from build123d import *

# Parameters (mm, degrees)
F0_R     = 2.5
F1_DEPTH = 3
F2_DEPTH = 5
F3_R     = 3
F3_R_2   = 2.5
F4_DEPTH = 2


with BuildPart() as f1:
    # F0 (on Top) → F1 (new body)
    with BuildSketch(Plane.XY):
        with BuildLine():
            Line((-28, 0), (0, 0))
            Line((0, 0), (0, 25))
            Line((0, 25), (-13, 25))
            ThreePointArc((-13, 25), (-16.3893239512, 24.6120663547), (-19.6033368631, 23.4683310871))
            ThreePointArc((-19.6033368631, 23.4683310871), (-18.0971524178, 22.6214718865), (-17.5, 21))
            ThreePointArc((-17.5, 21), (-20.3463811518, 18.5241122607), (-22.4040160781, 21.6860806776))
            ThreePointArc((-22.4040160781, 21.6860806776), (-25.1440747457, 18.8046265435), (-27.0307720104, 15.3044732813))
            ThreePointArc((-27.0307720104, 15.3044732813), (-25.9175651302, 14.3832805258), (-25.5, 13))
            ThreePointArc((-25.5, 13), (-26.2292882388, 11.235182769), (-27.991663887, 10.5000138982))
            ThreePointArc((-27.991663887, 10.5000138982), (-27.997915827, 10.2500416911), (-28, 10))
            Line((-28, 10), (-28, 7.5))
            ThreePointArc((-28, 7.5), (-26.232233047, 6.767766953), (-25.5, 5))
            ThreePointArc((-25.5, 5), (-26.232233047, 3.232233047), (-28, 2.5))
            Line((-28, 2.5), (-28, 0))
        make_face()
        with Locations((-20, 5)):
            Circle(F0_R, mode=Mode.SUBTRACT)
        with Locations((-12, 5)):
            Circle(F0_R, mode=Mode.SUBTRACT)
        with Locations((-4, 5)):
            Circle(F0_R, mode=Mode.SUBTRACT)
        with Locations((-20, 13)):
            Circle(F0_R, mode=Mode.SUBTRACT)
        with Locations((-12, 13)):
            Circle(F0_R, mode=Mode.SUBTRACT)
        with Locations((-4, 13)):
            Circle(F0_R, mode=Mode.SUBTRACT)
        with Locations((-12, 21)):
            Circle(F0_R, mode=Mode.SUBTRACT)
        with Locations((-4, 21)):
            Circle(F0_R, mode=Mode.SUBTRACT)
        with BuildLine():
            ThreePointArc((-17.5, 21), (-18.0971524178, 22.6214718865), (-19.6033368631, 23.4683310871))
            ThreePointArc((-19.6033368631, 23.4683310871), (-21.0531323829, 22.654922316), (-22.4040160781, 21.6860806776))
            ThreePointArc((-22.4040160781, 21.6860806776), (-20.3463811518, 18.5241122607), (-17.5, 21))
        make_face()
        with BuildLine():
            Line((0, 25), (0, 0))
            Line((0, 0), (28, 0))
            Line((28, 0), (28, 2.5))
            ThreePointArc((28, 2.5), (25.5, 5), (28, 7.5))
            Line((28, 7.5), (28, 10))
            ThreePointArc((28, 10), (27.997915827, 10.2500416911), (27.991663887, 10.5000138982))
            ThreePointArc((27.991663887, 10.5000138982), (25.5485483108, 12.5097096622), (27.0307720104, 15.3044732813))
            ThreePointArc((27.0307720104, 15.3044732813), (25.1440747457, 18.8046265435), (22.4040160781, 21.6860806776))
            ThreePointArc((22.4040160781, 21.6860806776), (22.4758877393, 21.3463811518), (22.5, 21))
            ThreePointArc((22.5, 21), (18.3785281135, 19.0971524178), (19.6033368631, 23.4683310871))
            ThreePointArc((19.6033368631, 23.4683310871), (16.3893239512, 24.6120663547), (13, 25))
            Line((13, 25), (0, 25))
        make_face()
        with Locations((4, 5)):
            Circle(F0_R, mode=Mode.SUBTRACT)
        with Locations((12, 5)):
            Circle(F0_R, mode=Mode.SUBTRACT)
        with Locations((20, 5)):
            Circle(F0_R, mode=Mode.SUBTRACT)
        with Locations((4, 13)):
            Circle(F0_R, mode=Mode.SUBTRACT)
        with Locations((12, 13)):
            Circle(F0_R, mode=Mode.SUBTRACT)
        with Locations((20, 13)):
            Circle(F0_R, mode=Mode.SUBTRACT)
        with Locations((4, 21)):
            Circle(F0_R, mode=Mode.SUBTRACT)
        with Locations((12, 21)):
            Circle(F0_R, mode=Mode.SUBTRACT)
        with BuildLine():
            ThreePointArc((22.4040160781, 21.6860806776), (21.0531323829, 22.654922316), (19.6033368631, 23.4683310871))
            ThreePointArc((19.6033368631, 23.4683310871), (18.3785281135, 19.0971524178), (22.5, 21))
            ThreePointArc((22.5, 21), (22.4758877393, 21.3463811518), (22.4040160781, 21.6860806776))
        make_face()
        with BuildLine():
            ThreePointArc((-27.0307720104, 15.3044732813), (-27.7087101354, 12.9417420271), (-27.991663887, 10.5000138982))
            ThreePointArc((-27.991663887, 10.5000138982), (-26.2292882388, 11.235182769), (-25.5, 13))
            ThreePointArc((-25.5, 13), (-25.9175651302, 14.3832805258), (-27.0307720104, 15.3044732813))
        make_face()
        with BuildLine():
            Line((-28, 7.5), (-28, 2.5))
            ThreePointArc((-28, 2.5), (-26.232233047, 3.232233047), (-25.5, 5))
            ThreePointArc((-25.5, 5), (-26.232233047, 6.767766953), (-28, 7.5))
        make_face()
        with BuildLine():
            ThreePointArc((28, 7.5), (25.5, 5), (28, 2.5))
            Line((28, 2.5), (28, 7.5))
        make_face()
        with BuildLine():
            ThreePointArc((27.991663887, 10.5000138982), (27.7087101354, 12.9417420271), (27.0307720104, 15.3044732813))
            ThreePointArc((27.0307720104, 15.3044732813), (25.5485483108, 12.5097096622), (27.991663887, 10.5000138982))
        make_face()
    extrude(amount=F1_DEPTH)

    # F0 (on Top) → F2 (join)
    with BuildSketch(Plane.XY):
        with Locations((-20, 13)):
            Circle(F0_R)
        with Locations((-20, 5)):
            Circle(F0_R)
        with Locations((-12, 5)):
            Circle(F0_R)
        with Locations((-12, 13)):
            Circle(F0_R)
        with Locations((-12, 21)):
            Circle(F0_R)
        with Locations((-4, 21)):
            Circle(F0_R)
        with Locations((-4, 13)):
            Circle(F0_R)
        with Locations((-4, 5)):
            Circle(F0_R)
        with Locations((4, 13)):
            Circle(F0_R)
        with Locations((4, 21)):
            Circle(F0_R)
        with Locations((4, 5)):
            Circle(F0_R)
        with Locations((12, 5)):
            Circle(F0_R)
        with Locations((12, 13)):
            Circle(F0_R)
        with Locations((12, 21)):
            Circle(F0_R)
        with Locations((20, 13)):
            Circle(F0_R)
        with Locations((20, 5)):
            Circle(F0_R)
    extrude(amount=F2_DEPTH)

    # F3 (on Top) → F4 (cut)
    with BuildSketch(Plane.XY):
        with BuildLine():
            Line((13, 23.5), (0, 23.5))
            Line((0, 23.5), (-13, 23.5))
            ThreePointArc((-13, 23.5), (-15.5473326534, 23.2574920838), (-18.0031470352, 22.5386809412))
            ThreePointArc((-18.0031470352, 22.5386809412), (-20.2891608484, 21.3630160664), (-22.3108832056, 19.7753492997))
            ThreePointArc((-22.3108832056, 19.7753492997), (-25.4086043388, 15.3175688394), (-26.5, 10))
            Line((-26.5, 10), (-26.5, 1.5))
            Line((-26.5, 1.5), (0, 1.5))
            Line((0, 1.5), (26.5, 1.5))
            Line((26.5, 1.5), (26.5, 7.3416876048))
            ThreePointArc((26.5, 7.3416876048), (21.0000404053, 8.9844298396), (26.4826520886, 10.6841729742))
            ThreePointArc((26.4826520886, 10.6841729742), (25.26982822, 15.6303921225), (22.3108832056, 19.7753492997))
            ThreePointArc((22.3108832056, 19.7753492997), (20.2891608484, 21.3630160664), (18.0031470352, 22.5386809412))
            ThreePointArc((18.0031470352, 22.5386809412), (15.5473326534, 23.2574920838), (13, 23.5))
        make_face()
        with Locations((-16, 9)):
            Circle(F3_R, mode=Mode.SUBTRACT)
        with Locations((-8, 9)):
            Circle(F3_R, mode=Mode.SUBTRACT)
        with Locations((0, 9)):
            Circle(F3_R, mode=Mode.SUBTRACT)
        with Locations((8, 9)):
            Circle(F3_R, mode=Mode.SUBTRACT)
        with Locations((16, 9)):
            Circle(F3_R, mode=Mode.SUBTRACT)
        with Locations((-16, 17)):
            Circle(F3_R, mode=Mode.SUBTRACT)
        with Locations((-8, 17)):
            Circle(F3_R, mode=Mode.SUBTRACT)
        with Locations((0, 17)):
            Circle(F3_R, mode=Mode.SUBTRACT)
        with Locations((8, 17)):
            Circle(F3_R, mode=Mode.SUBTRACT)
        with Locations((16, 17)):
            Circle(F3_R, mode=Mode.SUBTRACT)
        with BuildLine():
            ThreePointArc((26.5, 10), (26.4956623253, 10.342196438), (26.4826520886, 10.6841729742))
            ThreePointArc((26.4826520886, 10.6841729742), (21.0000404053, 8.9844298396), (26.5, 7.3416876048))
            Line((26.5, 7.3416876048), (26.5, 9))
            Line((26.5, 9), (26.5, 10))
        make_face()
        with Locations((24, 9)):
            Circle(F3_R_2, mode=Mode.SUBTRACT)
        with Locations((16, 9)):
            Circle(F3_R_2)
        with Locations((8, 9)):
            Circle(F3_R_2)
        with Locations((8, 17)):
            Circle(F3_R_2)
        with Locations((16, 17)):
            Circle(F3_R_2)
        with Locations((0, 9)):
            Circle(F3_R_2)
        with Locations((-8, 9)):
            Circle(F3_R_2)
        with Locations((-16, 9)):
            Circle(F3_R_2)
        with Locations((-16, 17)):
            Circle(F3_R_2)
        with Locations((-8, 17)):
            Circle(F3_R_2)
        with Locations((0, 17)):
            Circle(F3_R_2)
        with Locations((24, 9)):
            Circle(F3_R_2)
    extrude(amount=F4_DEPTH, mode=Mode.SUBTRACT)


solid = f1.part
The listing builds one solid part. Answer for the finished solid, in the listing's coordinates (mm). A direction names the side the tool comes from. Coordinates: 2 decimals unless noted, no trailing zeros. Loops run counter-clockwise (first coordinate to the right, second up) from the corner with the lowest first, then second, coordinate; pieces in that order, holes last.
1) Find section A-A on z = 4. Give the number of separate pieces and of enclosed holes in the cut face, then the cut area to 3 significant figures.
2) Determine the mould class of faces 1 (the face through (-2.66, 23.11, 3.99)), 2 (the face through (6, 19, 0)) for opening direction Y: pulls with the +Y half, pulls with the -Y half, needs draft (parallel to the pull), parting line crosses it, or undercut.
3) Flat-ended cylindrical pins translate along their axes: pin 1 Ø1 at (y, z) = (15.5, 2) entering from +X; pin 2 Ø3 at (x, y) = (-16, 17) entering from -Z; pin 3 Ø1 at (y, z) = (20.5, 2) entering from +X. Find the tip coordinate at first contact, or state that the pin passes through.
4) A tool of negligible diameter and unlimited length cuts with its end or side. For faces 3 (the face through (5.34, 23.11, 3.99)), 4 (the face through (4, 21, 5)), 5 (the face through (8, 17, 2)), from which of +Z, -Z, +X, -X, +Y, -Y can it reach the whole face along a straight path? Write none if from no direction.
5) Find the intervals of material crossed by L1, parallel to Y at x = 3.5, z = 1.5; L2, parallel to X at y = 20.5, z = 3.55; L3, parallel to Y at x = -8, z = 1.4, in increasing order.
6) Find section C-C on x = 8. Write down the section's boundary in (y, z).
Values:
1. separate pieces: 16
1. enclosed holes: 0
1. area: 314 mm2
2. face 1: undercut
2. face 2: needs draft
3. pin 1: stops at x = 27.14
3. pin 2: stops at z = 2
3. pin 3: stops at x = 24.18
4. face 3: +Z
4. face 4: +Z, +X, -X, +Y, -Y
4. face 5: -Z
5. L1: y = 0 to 1.5, 23.5 to 25
5. L2: x = -14.45 to -9.55, -6.45 to -1.55, 1.55 to 6.45, 9.55 to 14.45
5. L3: y = 0 to 1.5, 6 to 6.5, 11.5 to 12, 14 to 14.5, 19.5 to 20, 23.5 to 25
6. outline: (0, 0) - (1.5, 0) - (1.5, 2) - (6, 2) - (6, 0) - (6.5, 0) - (6.5, 2) - (11.5, 2) - (11.5, 0) - (12, 0) - (12, 2) - (14, 2) - (14, 0) - (14.5, 0) - (14.5, 2) - (19.5, 2) - (19.5, 0) - (20, 0) - (20, 2) - (23.5, 2) - (23.5, 0) - (25, 0) - (25, 3) - (0, 3) - close
